from build123d import *

# Parameters (mm, degrees)
F0_W     = 55
F0_H     = 14
F1_DEPTH = 4
F2_W     = 36
F2_H     = 2
F3_DEPTH = 6
F4_W     = 36
F4_H     = 14
F5_DEPTH = 2


with BuildPart() as f1:
    # F0 (on Top) → F1 (new body)
    with BuildSketch(Plane.XY):
        Rectangle(F0_W, F0_H)
        Polygon((-25.5, -4), (-25.5, 4), (-16.5, 4), (-16.5, 0), (-16.5, -4), align=None, mode=Mode.SUBTRACT)
    extrude(amount=F1_DEPTH)

    # F2 (on face) → F3 (join)
    with BuildSketch(Plane.XY.offset(4)):
        with Locations((9.5, -6)):
            Rectangle(F2_W, F2_H)
        with Locations((9.5, 6)):
            Rectangle(F2_W, F2_H)
    extrude(amount=F3_DEPTH)

    # F4 (on face) → F5 (join)
    with BuildSketch(Plane.XY.offset(10)):
        with Locations((9.5, 0)):
            Rectangle(F4_W, F4_H)
    extrude(amount=F5_DEPTH)


solid = f1.part
Geometry check sheet. Reference: the model listing, model coordinates, mm. A direction names the side the tool comes from. Give positions to 0.01 mm unless a question says otherwise; leave off trailing zeros. Loops run counter-clockwise (first coordinate to the right, second up) from the corner with the lowest first, then second, coordinate; pieces in that order, holes last. Notation, with made-up numbers: M 39.5,43.5 L 70.5,43.5 A20 ccw 70.5,56.5 Z; hole C 68.5,18.5 d4. An arc over 180 degrees is marked long. Answer as a JSON object with one key per item and string values. Group by question number.
Item 1: Sectioned sample at A-A on y = 1.75. Record the boundary of the cut face in (x, z), plus the area to 3 significant figures.
Item 2: Access from +Z, -Z, +X, -X, +Y, -Y to the whole of each face (thin tool, end or side, straight path). Record for faces 1 (the flat face through (27.5, 0, 3)), 2 (the flat face through (-8.5, 0, 11)), 3 (the flat face through (-27.5, 0, 2)), 4 (the flat face through (9, 0, 10)), 5 (the flat face through (-21, 4, 2)).
Item 3: Gauge pin test, flat ends, axial feed: pin 1 (4 mm diameter, centred on y = 0.5, z = 7.5, fed in from -X); pin 2 (6 mm diameter, centred on y = 2.5, z = 8, fed in from -X); pin 3 (8 mm diameter, centred on x = -13.5, y = 2.5, fed in from +Z). Record the tip position at first contact, or that the pin passes through.
Item 4: Material ranges on L1, parallel to X at y = -2, z = 2.5; L2, parallel to Y at x = -25, z = 3; L3, parallel to Y at x = -0.5, z = 6, recorded low to high.
Item 5: Sectioned sample at C-C on z = 4.75. Record the boundary of the cut face in (x, y).
Item 6: Mould release check, pull along Z, two halves, no side actions. Record for faces 6 (the flat face through (6, 7, 6)), 7 (the flat face through (0, 0, 4)), 8 (the flat face through (0, 0, 0)): pulls with the +Z half, pulls with the -Z half, needs draft (parallel to the pull), parting line crosses it, or undercut.
Item 7: Sectioned sample at B-B on x = -20.5. Record the boundary of the cut face in (y, z), plus the area to 3 significant figures.
Item 8: Sectioned sample at D-D on x = 9. Record the boundary of the cut face in (y, z), plus the area to 3 significant figures.
Findings below:
{
 "1": {"outline": "M -27.5,0 L -25.5,0 L -25.5,4 L -27.5,4 Z; M -16.5,0 L 27.5,0 L 27.5,4 L -16.5,4 Z; M -8.5,10 L 27.5,10 L 27.5,12 L -8.5,12 Z", "area": "256 mm2"},
 "2": {"face 1": "+Z, -Z, +X, +Y, -Y", "face 2": "+Z, -X, +Y, -Y", "face 3": "+Z, -Z, -X, +Y, -Y", "face 4": "+X, -X", "face 5": "+Z, -Z"},
 "3": {"pin 1": "through", "pin 2": "x = -8.5", "pin 3": "z = 4"},
 "4": {"L1": "-27.5 to -25.5, -16.5 to 27.5", "L2": "-7 to -4, 4 to 7", "L3": "-7 to -5, 5 to 7"},
 "5": {"outline": "M -8.5,-7 L 27.5,-7 L 27.5,-5 L -8.5,-5 Z; M -8.5,5 L 27.5,5 L 27.5,7 L -8.5,7 Z"},
 "6": {"face 6": "needs draft", "face 7": "undercut", "face 8": "pulls with the -Z half"},
 "7": {"outline": "M -7,0 L -4,0 L -4,4 L -7,4 Z; M 4,0 L 7,0 L 7,4 L 4,4 Z", "area": "24.0 mm2"},
 "8": {"outline": "M -7,0 L 7,0 L 7,12 L -7,12 Z; hole M -5,4 L 5,4 L 5,10 L -5,10 Z", "area": "108 mm2"}
}
